Read the model definition and answer for the solid it produces. Units are mm, in the model's axes. A direction names the side the tool comes from. Round coordinates to 2 decimals unless told otherwise and drop trailing zeros. Write each loop counter-clockwise with the first axis right and the second up, starting at its lowest first coordinate (ties: lowest second). Pieces come first, ordered by that corner, then holes. Notation, with made-up numbers: (25.25, 5) -> (34.25, 5) arc R15 ccw to (34.25, 34) -> close; hole circle Ø9 at (49, 18.5). An arc over 180 degrees is marked (long way). Return JSON: item names as keys, results as strings.
from build123d import *

# Parameters (mm, degrees)
ESQUISSE1_R              = 1.7
ESQUISSE1_R_2            = 14
ESQUISSE1_W              = 342.3
ESQUISSE1_H              = 506.843253
BOSS_EXTRU_1_DEPTH       = 8
ESQUISSE2_W              = 20
ESQUISSE2_H              = 8
ENL_V_MAT_EXTRU_1_DEPTH  = 10
ESQUISSE4_W              = 8.5
ESQUISSE4_H              = 15.5
ENL_V_MAT_EXTRU_2_DEPTH  = 10
ESQUISSE5_W              = 8.5
ESQUISSE5_H              = 15.5
ENL_V_MAT_EXTRU_3_DEPTH  = 10
ESQUISSE6_R              = 3.15
ESQUISSE6_R_2            = 2.65
ENL_V_MAT_EXTRU_4_DEPTH  = 10
BOSS_EXTRU_2_DEPTH       = 8
BOSS_EXTRU_3_DEPTH       = 8
BOSS_EXTRU_4_DEPTH       = 8
BOSS_EXTRU_5_DEPTH       = 8
ESQUISSE13_W             = 40.5
ESQUISSE13_H             = 8.5
ENL_V_MAT_EXTRU_6_DEPTH  = 10
ESQUISSE15_R             = 2.6
ENL_V_MAT_EXTRU_7_DEPTH  = 10
BOSS_EXTRU_6_DEPTH       = 8
CONG_1_R                 = 25
ESQUISSE17_R             = 4
ENL_V_MAT_EXTRU_8_DEPTH  = 10
ENL_V_MAT_EXTRU_9_DEPTH  = 10
ESQUISSE20_R             = 2.15
ENL_V_MAT_EXTRU_10_DEPTH = 30
ESQUISSE21_R             = 2.6
ENL_V_MAT_EXTRU_11_DEPTH = 11
ESQUISSE22_R             = 2.6
ENL_V_MAT_EXTRU_12_DEPTH = 10


with BuildPart() as part:
    # Esquisse1 → Boss.-Extru.1 (new body)
    with BuildSketch(Plane.XY):
        Polygon((40, -47), (-434.3, -47), (-434.3, 601.343253), (-331.846883663, 601.343253), (-314.526375587, 591.343253), (-78.820508076, 591.343253), (-61.5, 601.343253), (40, 601.343253), align=None)
        with Locations((-12.374368671, 12.374368671)):
            Circle(ESQUISSE1_R, mode=Mode.SUBTRACT)
        with Locations((12.374368671, 12.374368671)):
            Circle(ESQUISSE1_R, mode=Mode.SUBTRACT)
        with Locations((-12.374368671, -12.374368671)):
            Circle(ESQUISSE1_R, mode=Mode.SUBTRACT)
        with Locations((12.374368671, -12.374368671)):
            Circle(ESQUISSE1_R, mode=Mode.SUBTRACT)
        Circle(ESQUISSE1_R_2, mode=Mode.SUBTRACT)
        with Locations((-197.15, 252.4216265)):
            Rectangle(ESQUISSE1_W, ESQUISSE1_H, mode=Mode.SUBTRACT)
    extrude(amount=BOSS_EXTRU_1_DEPTH)

    # Esquisse2 → Enlèv. mat.-Extru.1 (cut)
    with BuildSketch(Plane.XY.offset(8)):
        with Locations((-254.3, 532)):
            Rectangle(ESQUISSE2_W, ESQUISSE2_H)
        with Locations((-374.3, 532)):
            Rectangle(ESQUISSE2_W, ESQUISSE2_H)
        with Locations((-134.3, 532)):
            Rectangle(ESQUISSE2_W, ESQUISSE2_H)
        with Locations((-14.3, 532)):
            Rectangle(ESQUISSE2_W, ESQUISSE2_H)
    extrude(amount=-ENL_V_MAT_EXTRU_1_DEPTH, mode=Mode.SUBTRACT)

    # Esquisse4 → Enlèv. mat.-Extru.2 (cut)
    with BuildSketch(Plane.XY.offset(8)):
        with Locations((32, -36.5)):
            Rectangle(ESQUISSE4_W, ESQUISSE4_H)
        with Locations((32, 128.5)):
            Rectangle(ESQUISSE4_W, ESQUISSE4_H)
        with Locations((32, 293.5)):
            Rectangle(ESQUISSE4_W, ESQUISSE4_H)
        with Locations((32, 458.5)):
            Rectangle(ESQUISSE4_W, ESQUISSE4_H)
        with Locations((32, 563.5)):
            Rectangle(ESQUISSE4_W, ESQUISSE4_H)
    extrude(amount=-ENL_V_MAT_EXTRU_2_DEPTH, mode=Mode.SUBTRACT)

    # Esquisse5 → Enlèv. mat.-Extru.3 (cut)
    with BuildSketch(Plane.XY.offset(8)):
        with Locations((-426.3, 458.5)):
            Rectangle(ESQUISSE5_W, ESQUISSE5_H)
        with Locations((-426.3, 293.5)):
            Rectangle(ESQUISSE5_W, ESQUISSE5_H)
        with Locations((-426.3, 128.5)):
            Rectangle(ESQUISSE5_W, ESQUISSE5_H)
        with Locations((-426.3, -36.5)):
            Rectangle(ESQUISSE5_W, ESQUISSE5_H)
        with Locations((-426.3, 563.5)):
            Rectangle(ESQUISSE5_W, ESQUISSE5_H)
    extrude(amount=-ENL_V_MAT_EXTRU_3_DEPTH, mode=Mode.SUBTRACT)

    # Esquisse6 → Enlèv. mat.-Extru.4 (cut)
    with BuildSketch(Plane.XY.offset(8)):
        with Locations((-402.5, 83.4)):
            Circle(ESQUISSE6_R)
        with Locations((-402.5, 43.4)):
            Circle(ESQUISSE6_R)
        with Locations((-391.438608853, 124.84)):
            Circle(ESQUISSE6_R_2)
        with Locations((-411.438608853, 124.84)):
            Circle(ESQUISSE6_R_2)
    extrude(amount=-ENL_V_MAT_EXTRU_4_DEPTH, mode=Mode.SUBTRACT)

    # Esquisse8 → Boss.-Extru.2 (add)
    with BuildSketch(Plane.XY.offset(8)):
        Polygon((-26, -1), (-74, -1), (-74, 77), (-26, 129), align=None)
        Polygon((-368.3, 29), (-368.3, -1), (-74, -1), align=None)
        Polygon((-368.3, 475.843253), (-126, 505.843253), (-368.3, 505.843253), align=None)
    extrude(amount=-BOSS_EXTRU_2_DEPTH)

    # Esquisse9 → Boss.-Extru.3 (add)
    with BuildSketch(Plane.XY.offset(8)):
        Polygon((-434.3, -47), (-434.3, -53), (-329.3, -87), (-64, -87), (40, -62), (40, -47), align=None)
        with BuildLine():
            Line((-236.65, -62), (-156.65, -62))
            ThreePointArc((-156.65, -62), (-149.15, -69.5), (-156.65, -77))
            Line((-156.65, -77), (-236.65, -77))
            ThreePointArc((-236.65, -77), (-244.15, -69.5), (-236.65, -62))
        make_face(mode=Mode.SUBTRACT)
    extrude(amount=-BOSS_EXTRU_3_DEPTH)

    # Esquisse11 → Boss.-Extru.4 (add)
    with BuildSketch(Plane(origin=(0, 0, 0), x_dir=(-1, 0, 0), z_dir=(0, 0, -1))):
        Polygon((-40, -62), (-117, -43.490384615), (-117, 54.509615385), (-59.554373535, 94.509615385), (-40, 194.509615385), align=None)
    extrude(amount=-BOSS_EXTRU_4_DEPTH)

    # Esquisse14 → Boss.-Extru.5 (add)
    with BuildSketch(Plane.XY.offset(8)):
        Polygon((26.5, -65.245192308), (117, -65.245192308), (117, -43.490384615), align=None)
    extrude(amount=-BOSS_EXTRU_5_DEPTH)

    # Esquisse13 → Enlèv. mat.-Extru.6 (cut)
    with BuildSketch(Plane.XY.offset(8)):
        with Locations((92, -52)):
            Rectangle(ESQUISSE13_W, ESQUISSE13_H)
    extrude(amount=-ENL_V_MAT_EXTRU_6_DEPTH, mode=Mode.SUBTRACT)

    # Esquisse15 → Enlèv. mat.-Extru.7 (cut)
    with BuildSketch(Plane.XY.offset(8)):
        with Locations((-414.438608853, 378)):
            Circle(ESQUISSE15_R)
        with Locations((-414.438608853, 400)):
            Circle(ESQUISSE15_R)
        with Locations((18, 400)):
            Circle(ESQUISSE15_R)
        with Locations((18, 378)):
            Circle(ESQUISSE15_R)
    extrude(amount=-ENL_V_MAT_EXTRU_7_DEPTH, mode=Mode.SUBTRACT)

    # Esquisse16 → Boss.-Extru.6 (add)
    with BuildSketch(Plane.XY.offset(8)):
        Polygon((117, 54.509615385), (150, 31.531364798), (150, -65.245192308), (117, -65.245192308), align=None)
    extrude(amount=-BOSS_EXTRU_6_DEPTH)

    # Congé1
    cong_1_edges = [part.edges().sort_by_distance(p)[0] for p in [
        (150, 31.531364798, 4),
        (150, -65.245192308, 4),
    ]]
    fillet(cong_1_edges, radius=CONG_1_R)

    # Esquisse17 → Enlèv. mat.-Extru.8 (cut)
    with BuildSketch(Plane.XY.offset(8)):
        with Locations((-404.438608853, 586.343252998)):
            Circle(ESQUISSE17_R)
        with Locations((-374.438608853, 586.343252998)):
            Circle(ESQUISSE17_R)
        with Locations((-22, 586.343253)):
            Circle(ESQUISSE17_R)
        with Locations((8, 586.343253)):
            Circle(ESQUISSE17_R)
    extrude(amount=-ENL_V_MAT_EXTRU_8_DEPTH, mode=Mode.SUBTRACT)

    # Esquisse19 → Enlèv. mat.-Extru.9 (cut)
    with BuildSketch(Plane.XY.offset(8)):
        with BuildLine():
            Line((110, -17.345192308), (105, -17.345192308))
            ThreePointArc((105, -17.345192308), (102.9, -15.245192308), (105, -13.145192308))
            Line((105, -13.145192308), (110, -13.145192308))
            ThreePointArc((110, -13.145192308), (112.1, -15.245192308), (110, -17.345192308))
        make_face()
        with BuildLine():
            Line((80, -13.115192308), (85, -13.115192308))
            ThreePointArc((85, -13.115192308), (87.13, -15.245192308), (85, -17.375192308))
            Line((85, -17.375192308), (80, -17.375192308))
            ThreePointArc((80, -17.375192308), (77.87, -15.245192308), (80, -13.115192308))
        make_face()
        with BuildLine():
            Line((110, 12.654807692), (105, 12.654807692))
            ThreePointArc((105, 12.654807692), (102.9, 14.754807692), (105, 16.854807692))
            Line((105, 16.854807692), (110, 16.854807692))
            ThreePointArc((110, 16.854807692), (112.1, 14.754807692), (110, 12.654807692))
        make_face()
        with BuildLine():
            Line((80, 16.854807692), (85, 16.854807692))
            ThreePointArc((85, 16.854807692), (87.1, 14.754807692), (85, 12.654807692))
            Line((85, 12.654807692), (80, 12.654807692))
            ThreePointArc((80, 12.654807692), (77.9, 14.754807692), (80, 16.854807692))
        make_face()
    extrude(amount=-ENL_V_MAT_EXTRU_9_DEPTH, mode=Mode.SUBTRACT)

    # Esquisse20 → Enlèv. mat.-Extru.10 (cut)
    with BuildSketch(Plane.XY.offset(8)):
        with Locations((-21.5, 194.843253)):
            Circle(ESQUISSE20_R)
        with Locations((-21.5, 364.843253)):
            Circle(ESQUISSE20_R)
        with Locations((-67, 510.343253)):
            Circle(ESQUISSE20_R)
        with Locations((-257.3, 494.120907239)):
            Circle(ESQUISSE20_R)
        with Locations((-372.8, 410.870792038)):
            Circle(ESQUISSE20_R)
        with Locations((-372.8, 260.870792038)):
            Circle(ESQUISSE20_R)
        with Locations((-372.8, 130.870792038)):
            Circle(ESQUISSE20_R)
        with Locations((-325, 20.062817018)):
            Circle(ESQUISSE20_R)
        with Locations((-145, 1.714193165)):
            Circle(ESQUISSE20_R)
    extrude(amount=-ENL_V_MAT_EXTRU_10_DEPTH, mode=Mode.SUBTRACT)

    # Esquisse21 → Enlèv. mat.-Extru.11 (cut)
    with BuildSketch(Plane(origin=(0, 0, 0), x_dir=(-1, 0, 0), z_dir=(0, 0, -1))):
        with Locations((47, -43)):
            Circle(ESQUISSE21_R)
        with Locations((27, -43)):
            Circle(ESQUISSE21_R)
        with Locations((367.3, -43)):
            Circle(ESQUISSE21_R)
        with Locations((347.3, -43)):
            Circle(ESQUISSE21_R)
    extrude(amount=-ENL_V_MAT_EXTRU_11_DEPTH, mode=Mode.SUBTRACT)

    # Esquisse22 → Enlèv. mat.-Extru.12 (cut)
    with BuildSketch(Plane(origin=(0, 0, 0), x_dir=(-1, 0, 0), z_dir=(0, 0, -1))):
        with Locations((-18, 232)):
            Circle(ESQUISSE22_R)
        with Locations((-18, 210)):
            Circle(ESQUISSE22_R)
        with Locations((414.438608853, 232)):
            Circle(ESQUISSE22_R)
        with Locations((414.438608853, 210)):
            Circle(ESQUISSE22_R)
    extrude(amount=-ENL_V_MAT_EXTRU_12_DEPTH, mode=Mode.SUBTRACT)


solid = part.part
Item 1: A tool of negligible diameter and unlimited length cuts with its end or side. For faces 4 (the flat face through (-8, 262, 0)), 5 (the flat face through (-219.09, 13.79, 4.06)), from which of +Z, -Z, +X, -X, +Y, -Y can it reach the whole face along a straight path? Write none if from no direction.
Worked answers:
{"face 4": "-Z, +X, -X, +Y, -Y", "face 5": "+Z, -Z"}
Item 2: Section B-B (x = -228.5) is taken. Give the vertices of the cut face in (y, z).
Worked answers:
{"outline": "(-87, 0) -> (-77, 0) -> (-77, 8) -> (-87, 8) -> close; (-62, 0) -> (14.75, 0) -> (14.75, 8) -> (-62, 8) -> close; (493.15, 0) -> (591.34, 0) -> (591.34, 8) -> (493.15, 8) -> close"}
Item 3: For a pull along Y with two mould halves and no side action, classify faces 1 (the flat face through (-248.846, 490.633, 4.056)), 2 (the flat face through (-19.384, -76.275, 4.056)), 3 (the flat face through (49.914, 143.81, 3.944)) as released by +Y, released by -Y, zero draft, split by the parting line, or undercut.
Worked answers:
{"face 1": "undercut", "face 2": "released by -Y", "face 3": "released by +Y"}
Item 4: Straight lines are drawn through the part: L1, parallel to X at y = 316, z = 7.5; L2, parallel to Y at x = -170.5, z = 5; L3, parallel to Y at x = -126, z = 7. For each, find the intervals that lie inside material, in ascending order. Write a range as [from, to].
Worked answers:
{"L1": "x = [-434.3, -368.3], [-26, 40]", "L2": "y = [-87, -77], [-62, 8.84], [500.33, 591.34]", "L3": "y = [-87, 4.3], [505.84, 528], [536, 591.34]"}
Item 5: Section A-A (y = 177.5) is taken. Give the vertices of the cut face in (x, z).
Worked answers:
{"outline": "(-434.3, 0) -> (-368.3, 0) -> (-368.3, 8) -> (-434.3, 8) -> close; (-26, 0) -> (43.33, 0) -> (43.33, 8) -> (-26, 8) -> close"}
Item 6: Section D-D (x = 50) is taken. Give the vertices of the cut face in (y, z), then the cut area to 3 significant figures.
Worked answers:
{"outline": "(-65.25, 0) -> (143.37, 0) -> (143.37, 8) -> (-65.25, 8) -> close", "area": "1,670 mm2"}
Item 7: Section C-C (z = 5.5) is taken. State how many separate pieces and enclosed holes the cut face has, then the cut area to 3 significant figures.
Worked answers:
{"separate pieces": "1", "enclosed holes": "55", "area": "171,000 mm2"}
Item 8: Flat-ended cylindrical pins translate along their axes: pin 1 (4 mm diameter, centred on y = 98.5, z = 3.5, fed in from +X); pin 2 (10 mm diameter, centred on x = -35, y = 440, fed in from +Z); pin 3 (1.5 mm diameter, centred on y = 303, z = 2, fed in from +X); pin 4 (4 mm diameter, centred on y = -52, z = 5.5, fed in from +X). Find the tip coordinate at first contact, or state that the pin passes through.
Worked answers:
{"pin 1": "stops at x = 59.17", "pin 2": "passes through", "pin 3": "stops at x = 40", "pin 4": "stops at x = 148.02"}
